from build123d import *

# Parameters (mm, degrees)
ESBO_O1_W                = 93
ESBO_O1_H                = 50
RESSALTO_EXTRUS_O1_DEPTH = 1.26
ESBO_O2_W                = 1.26
ESBO_O2_H                = 47.48
RESSALTO_EXTRUS_O2_DEPTH = 1.26
ESBO_O3_W                = 10
ESBO_O3_H                = 1.26
RESSALTO_EXTRUS_O3_DEPTH = 2.26
CORTE_EXTRUS_O1_DEPTH    = 1.26
ESBO_O5_W                = 66.74
ESBO_O5_H                = 3.26
RESSALTO_EXTRUS_O4_DEPTH = 2
CORTE_EXTRUS_O3_DEPTH    = 72


with BuildPart() as part:
    # Esboço1 → Ressalto-extrusão1 (new body)
    with BuildSketch(Plane(origin=(0, 0, 0), x_dir=(1, 0, 0), z_dir=(0, 1, 0))):
        with Locations((46.5, 25)):
            Rectangle(ESBO_O1_W, ESBO_O1_H)
    extrude(amount=RESSALTO_EXTRUS_O1_DEPTH)

    # Esboço2 → Ressalto-extrusão2 (add)
    with BuildSketch(Plane(origin=(0, 1.26, 0), x_dir=(1, 0, 0), z_dir=(0, 1, 0))):
        with Locations((0.63, 25)):
            Rectangle(ESBO_O2_W, ESBO_O2_H)
    extrude(amount=RESSALTO_EXTRUS_O2_DEPTH)

    # Esboço3 → Ressalto-extrusão3 (add)
    with BuildSketch(Plane(origin=(0, 1.26, 0), x_dir=(1, 0, 0), z_dir=(0, 1, 0))):
        with Locations((6.26, 25.5)):
            Rectangle(ESBO_O3_W, ESBO_O3_H)
    extrude(amount=RESSALTO_EXTRUS_O3_DEPTH)

    # Esboço4 → Corte-extrusão1 (cut)
    with BuildSketch(Plane.XY.offset(-24.87)):
        with BuildLine():
            Line((1.26, 3.52), (11.26, 3.52))
            Line((11.26, 3.52), (11.26, 1.26))
            ThreePointArc((11.26, 1.26), (6.158122993, 1.939216781), (1.26, 3.52))
        make_face()
    extrude(amount=-CORTE_EXTRUS_O1_DEPTH, mode=Mode.SUBTRACT)

    # Esboço5 → Ressalto-extrusão4 (add)
    with BuildSketch(Plane(origin=(0, 1.26, 0), x_dir=(1, 0, 0), z_dir=(0, 1, 0))):
        with Locations((58.37, 2.89)):
            Rectangle(ESBO_O5_W, ESBO_O5_H)
        with Locations((58.37, 47.11)):
            Rectangle(ESBO_O5_W, ESBO_O5_H)
    extrude(amount=RESSALTO_EXTRUS_O4_DEPTH)

    # Esboço6 → Corte-extrusão3 (cut)
    with BuildSketch(Plane(origin=(91.74, 0, 0), x_dir=(0, 0, -1), z_dir=(1, 0, 0))):
        Polygon((3.262223764, 1.26), (1.26, 3.26), (1.26, 1.26), align=None)
        Polygon((46.737776236, 1.26), (48.74, 3.26), (48.74, 1.26), align=None)
    extrude(amount=-CORTE_EXTRUS_O3_DEPTH, mode=Mode.SUBTRACT)


solid = part.part
Work out the finished part from the listing and answer in its coordinate system (mm). A direction names the side the tool comes from. Coordinates: 2 decimals unless noted, no trailing zeros. Write each loop counter-clockwise with the first axis right and the second up, starting at its lowest first coordinate (ties: lowest second). Pieces come first, ordered by that corner, then holes.
1. The part is cut by section C-C, the plane z = -42. Write down the section's boundary in (x, y), and give its area (3 significant figures).
Results list:
outline: (0, 0) - (93, 0) - (93, 1.26) - (1.26, 1.26) - (1.26, 2.52) - (0, 2.52) - close
area: 119 mm2
2. Flat-ended cylindrical pins translate along their axes: pin 1 (1.6 mm diameter, centred on x = 73.5, y = 2.5, fed in from -Z); pin 2 (2 mm diameter, centred on y = 2.5, z = -2.5, fed in from +X); pin 3 (10 mm diameter, centred on x = 78.5, z = -6, fed in from +Y). Find the tip coordinate at first contact, or state that the pin passes through.
Results list:
pin 1: stops at z = -48.74
pin 2: stops at x = 91.74
pin 3: stops at y = 3.26
3. The part is cut by section A-A, the plane x = 63. Write down the section's boundary in (y, z), and give its area (3 significant figures).
Results list:
outline: (0, -50) - (1.26, -50) - (1.26, -46.74) - (3.26, -48.74) - (3.26, -45.48) - (1.26, -45.48) - (1.26, -4.52) - (3.26, -4.52) - (3.26, -1.26) - (1.26, -3.26) - (1.26, 0) - (0, 0) - close
area: 72.0 mm2
4. The part is cut by section B-B, the plane y = 1.9. Write down the section's boundary in (x, z).
Results list:
outline: (0, -48.74) - (1.26, -48.74) - (1.26, -26.13) - (6.33, -26.13) - (6.33, -24.87) - (1.26, -24.87) - (1.26, -1.26) - (0, -1.26) - close; (25, -47.38) - (91.74, -47.38) - (91.74, -45.48) - (25, -45.48) - close; (25, -4.52) - (91.74, -4.52) - (91.74, -2.62) - (25, -2.62) - close
5. For faces 1 (the flat face through (4, 2, -24.87)), 2 (the flat face through (91.74, 2, -47)), 3 (the flat face through (25, 2, -47)), determine the directions among +Z, -Z, +X, -X, +Y, -Y from which every point of the face is accessible in a straight line to the end or side of a thin tool.
Results list:
face 1: +Z, +X, +Y
face 2: +Z, -Z, +X, +Y
face 3: +Z, -Z, +Y
6. Consider line 1 along Y through (x, z) = (50, -20.5); line 2 along Y through (x, z) = (51, -46). Determine where each line is inside the solid, lowest interval first.
Results list:
line 1: y = 0 to 1.26
line 2: y = 0 to 3.26
7. For a pull along Z with two mould halves and no side action, classify faces 4 (the flat face through (25, 2, -3)), 5 (the flat face through (58, 2, -4.52)), 6 (the flat face through (46, 1.26, -25)), 7 (the flat face through (4, 2, -26.13)) as +Z half, -Z half, draft (parallel to the pull), parting line (faces both ways), or undercut.
Results list:
face 4: draft
face 5: undercut
face 6: undercut
face 7: -Z half
